from build123d import *

# Parameters (mm, degrees)
BODYSKE_R       = 0.825
BODYSKE_R_2     = 0.425
BODY_DEPTH      = 41
HOLE_PROFILE_R  = 0.8
CUT1_DEPTH      = 0.825
CUT1_DEPTH_BACK = 42.54816492
CUT2_DEPTH      = 42.548164932
FILLET_2_R      = 1


with BuildPart() as part:
    # BodySke → Body (new body)
    with BuildSketch(Plane.XY):
        with BuildLine():
            Line((4.165063509, -1.25), (3, -3.267949192))
            ThreePointArc((3, -3.267949192), (0, -5), (-3, -3.267949192))
            Line((-3, -3.267949192), (-4.165063509, -1.25))
            ThreePointArc((-4.165063509, -1.25), (-4.283863644, 1.016841608), (-2.519779227, 2.445369002))
            Line((-2.519779227, 2.445369002), (-0.606233769, 2.852105645))
            ThreePointArc((-0.606233769, 2.852105645), (0, 2.915823382), (0.606233769, 2.852105645))
            Line((0.606233769, 2.852105645), (2.519779227, 2.445369002))
            ThreePointArc((2.519779227, 2.445369002), (4.283863644, 1.016841608), (4.165063509, -1.25))
        make_face()
        Circle(BODYSKE_R, mode=Mode.SUBTRACT)
        with Locations((-3, 0)):
            Circle(BODYSKE_R_2, mode=Mode.SUBTRACT)
        with Locations((3, 0)):
            Circle(BODYSKE_R_2, mode=Mode.SUBTRACT)
        with Locations((0, -3)):
            Circle(BODYSKE_R_2, mode=Mode.SUBTRACT)
    extrude(amount=BODY_DEPTH)

    # Hole: sweep along a path in HoleSke
    with BuildLine() as hole_path:  # in the path sketch's own coordinates; laid on its plane below (add() does not lay a ready-made edge on the line's plane)
        Line((6, 2.915823382), (6, 1.704499781))
        add(Edge.make_bspline(
            [(6, 1.704499781), (6, 0.035966381), (4.619948081, 0), (0, 0)],
            knots=[0, 0, 0, 0, 1, 1, 1, 1], degree=3))
    # Hole profile (on start of the path) → Hole (sweep, cut)
    with BuildSketch(Plane(origin=(-0.606233769, 2.852105645, 6), x_dir=(-0.9781476007338055, -0.2079116908177599, 0), z_dir=(0.2079116908177599, -0.9781476007338055, 0))):
        Circle(HOLE_PROFILE_R)
    sweep(path=Plane(origin=(0, 0, 0), x_dir=(0, 0, 1), z_dir=(-0.9781476007338055, -0.2079116908177599, 0)) * hole_path.line, mode=Mode.SUBTRACT)

    # Cut1Ske → Cut1 (cut, two sides: drawn at the far end of the back side and taken through both)
    with BuildSketch(Plane(origin=(0, 0, 0), x_dir=(1, 0, 0), z_dir=(0, 1, 0)).offset(-CUT1_DEPTH_BACK)):
        with BuildLine():
            Line((1.75, -9.5), (1.75, -36))
            ThreePointArc((1.75, -36), (0, -37.75), (-1.75, -36))
            Line((-1.75, -36), (-1.75, -9.5))
            ThreePointArc((-1.75, -9.5), (0, -7.75), (1.75, -9.5))
        make_face()
    extrude(amount=CUT1_DEPTH + CUT1_DEPTH_BACK, mode=Mode.SUBTRACT)

    # Cut2Ske → Cut2 (cut, through all)
    with BuildSketch(Plane(origin=(0, 0, 0), x_dir=(1, 0, 0), z_dir=(0, 1, 0))):
        with BuildLine():
            Line((-1.75, -20.25), (-1.75, -9.5))
            ThreePointArc((-1.75, -9.5), (0, -7.75), (1.75, -9.5))
            Line((1.75, -9.5), (1.75, -20.25))
            ThreePointArc((1.75, -20.25), (0, -22), (-1.75, -20.25))
        make_face()
        with BuildLine():
            Line((1.75, -25.25), (1.75, -36))
            ThreePointArc((1.75, -36), (0, -37.75), (-1.75, -36))
            Line((-1.75, -36), (-1.75, -25.25))
            ThreePointArc((-1.75, -25.25), (0, -23.5), (1.75, -25.25))
        make_face()
    extrude(amount=CUT2_DEPTH, mode=Mode.SUBTRACT)

    # Fillet 2
    fillet_2_edges = [part.edges().sort_by_distance(p)[0] for p in [
        (-1.75, 0.825, 22.75),
        (1.75, 0.825, 22.75),
    ]]
    fillet(fillet_2_edges, radius=FILLET_2_R)


solid = part.part
Source: CAD feature listing. Evaluate the final solid. Frame: model axes, mm. A direction names the side the tool comes from. Round coordinates to 2 decimals unless told otherwise and drop trailing zeros. Loops run counter-clockwise (first coordinate to the right, second up) from the corner with the lowest first, then second, coordinate; pieces in that order, holes last. Notation, with made-up numbers: M -30.75,-3.75 L -5.75,-3.75 A5 cw -5.75,1.25 Z; hole C -40,18.5 d10. An arc over 180 degrees is marked long. Return JSON: item names as keys, results as strings. Group by question number.
1. Section query B-B on x = 0. State how many separate pieces and enclosed holes the cut face has, and give its area (3 significant figures).
2. Section query A-A on z = 10. Output: boundary loops of the cut face in (x, y) (3 decimals).
3. Reachability of faces 4 (the face through (-0.04, -1.1, 7.75)), 5 (the face through (-2.19, -4.22, 20.21)) from +Z, -Z, +X, -X, +Y, -Y: full face, straight path, thin tool, end or side. Return the list, or none.
4. Material intervals for line 1 along Y through (x, z) = (0, 40) (3 decimals); line 2 along Z through (x, y) = (0, 2.5); line 3 along Y through (x, z) = (0, 4) (3 decimals), sorted ascending. Write a range as from..to.
5. Pin query (flat end, axial travel): pin 1 (2 mm diameter, centred on x = -1, z = 34, fed in from -Y); pin 2 (1.7 mm diameter, centred on x = 0.5, z = 22.5, fed in from -Y) (3 decimals); pin 3 (1 mm diameter, centred on x = 0, y = 0, fed in from -Z). Return the tip coordinate at first contact, or that it passes through.
6. Mould query, pull axis X, two halves, no side actions, for faces 1 (the face through (-4.297, 0.987, 20.213)), 2 (the face through (-1.2, 2.1, 6.31)), 3 (the face through (-0.009, 2.916, 39.297)). Classes: released by +X, released by -X, zero draft, split by the parting line, or undercut.
Checks:
{
 "1": {"separate pieces": "8", "enclosed holes": "0", "area": "59.6 mm²"},
 "2": {"outline": "M -4.165,-1.25 L -3,-3.268 A3.464 ccw -1.75,-4.525 L -1.75,2.609 L -2.52,2.445 A2.5 ccw Z; M 1.75,-4.525 A3.464 ccw 3,-3.268 L 4.165,-1.25 A2.5 ccw 2.52,2.445 L 1.75,2.609 Z; hole C -3,0 d0.85; hole C 3,0 d0.85"},
 "3": {"face 4": "+Y, -Y", "face 5": "+Z, -Z, -Y"},
 "4": {"line 1": "y = -5..-3.425, -2.575..-0.825, 0.825..2.916", "line 2": "z = 0..5.39, 6.61..7.75, 22..23.5, 37.75..41", "line 3": "y = -5..-3.425, -2.575..-0.825, 0.909..2.916"},
 "5": {"pin 1": "stops at y = -4.53", "pin 2": "stops at y = 0.625", "pin 3": "passes through"},
 "6": {"face 1": "released by -X", "face 2": "undercut", "face 3": "split by the parting line"}
}
